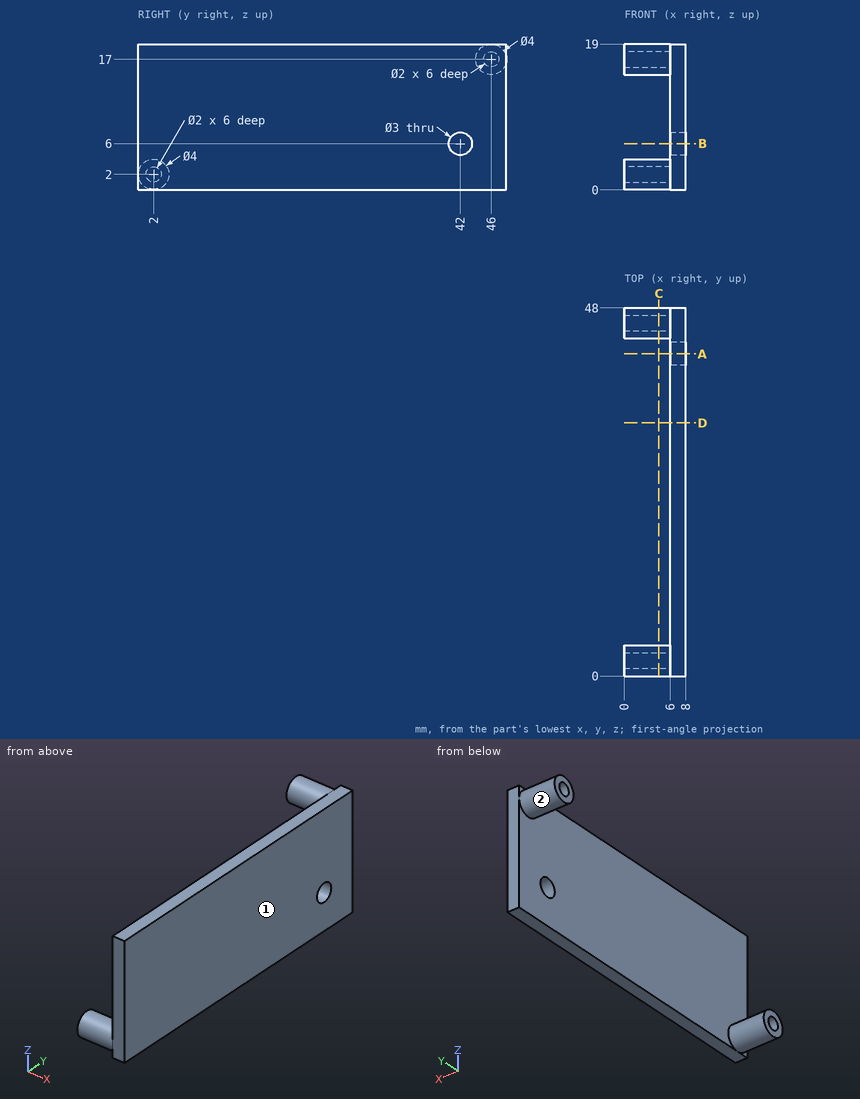
Could you check a few things on this drawing? It's one solid part, dimensions in mm from its lowest x, y, z. A direction names the side the tool comes from. Coordinates: 2 decimals unless noted, no trailing zeros. Order: outer loops, then holes, each group sorted by start corner. A loop starts at its lowest first (then second) coordinate and runs counter-clockwise, first axis right, second up.
1) Imagine slicing it at A-A on y = 42. List the corners of the cut face in (x, z) for me.
2) Imagine slicing it at B-B on z = 6. List the corners of the cut face in (x, y) for me, and give its area (3 significant figures).
3) Imagine slicing it at C-C on x = 4.5. List the corners of the cut face in (y, z) for me, and give its area (3 significant figures).
4) Imagine slicing it at D-D on y = 33. List the corners of the cut face in (x, z) for me, and give its area (3 significant figures).
5) Will these pins go through, and if not, where does the flat tip stop? pin 1 (3 mm diameter, centred on x = 5.5, y = 24, fed in from -Z); pin 2 (1 mm diameter, centred on y = 15, z = 13.5, fed in from -X).
6) Which directions (+Z, -Z, +X, -X, +Y, -Y) give clear straight access to the entire face, cutting with the end or side of a thin tool? Please do the marked faces 1 and 2.
7) I need wall thicknesses on line 1 (Y direction, x = 7.4, z = 6); line 2 (Y direction, x = 1.6, z = 2); line 3 (X direction, y = 14.5, z = 8). Which ranges of each line are inside material? Lowest first, please.
Response values:
1. outline: (6, 0) - (8, 0) - (8, 4.5) - (6, 4.5) - close; (6, 7.5) - (8, 7.5) - (8, 19) - (6, 19) - close
2. outline: (6, 0) - (8, 0) - (8, 40.5) - (6, 40.5) - close; (6, 43.5) - (8, 43.5) - (8, 48) - (6, 48) - close
2. area: 90.0 mm2
3. outline: circle Ø4 at (2, 2); circle Ø4 at (46, 17); hole circle Ø2 at (2, 2); hole circle Ø2 at (46, 17)
3. area: 18.8 mm2
4. outline: (6, 0) - (8, 0) - (8, 19) - (6, 19) - close
4. area: 38.0 mm2
5. pin 1: stops at z = 0
5. pin 2: stops at x = 6
6. face 1: +Z, -Z, +X, +Y, -Y
6. face 2: -X
7. line 1: y = 0 to 40.5, 43.5 to 48
7. line 2: y = 0 to 1, 3 to 4
7. line 3: x = 6 to 8
